Input: part model. Units: mm. Frame: model coordinates. Give positions to 0.01 mm unless a question says otherwise; leave off trailing zeros. Write each loop counter-clockwise with the first axis right and the second up, starting at its lowest first coordinate (ties: lowest second). Pieces come first, ordered by that corner, then holes. Notation, with made-up numbers: (33.5, 4.5) - (70.5, 4.5) arc R25 cw to (70.5, 35.5) - close; hole circle Ø8 at (65, -6). An arc over 180 degrees is marked (long way). Answer as CSV lines item,"result".
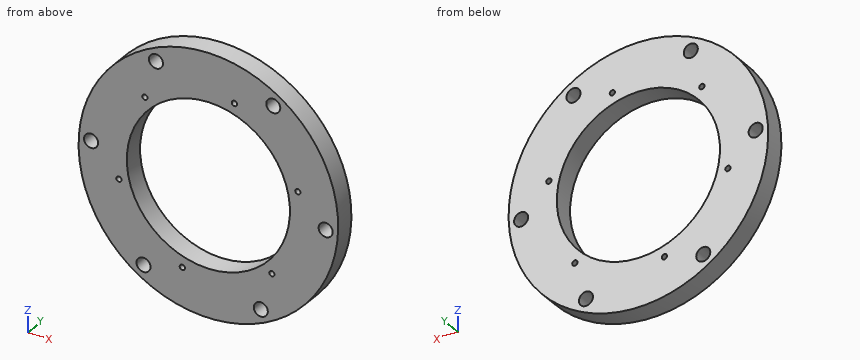
```python
from build123d import *

# Parameters (mm, degrees)
SKETCH_1_R      = 74
SKETCH_1_R_2    = 46.5
SKETCH_1_R_3    = 1.5
SKETCH_1_R_4    = 4
EXTRUDE_2_DEPTH = 12


with BuildPart() as part:
    # 草图1 → 凸台-拉伸2 (new body)
    with BuildSketch(Plane(origin=(0, 0, 0), x_dir=(1, 0, 0), z_dir=(0, 1, 0))):
        with Locations(Location((0, 0, 0), (0, 0, 270))):
            Circle(SKETCH_1_R)
        with Locations(Location((0, 0, 0), (0, 0, 270))):
            Circle(SKETCH_1_R_2, mode=Mode.SUBTRACT)
        with Locations(Location((36.199702934, 38.024091146, 0), (0, 0, 270))):
            Circle(SKETCH_1_R_3, mode=Mode.SUBTRACT)
        with Locations(Location((29.881416045, 59.967499324, 0), (0, 0, 270))):
            Circle(SKETCH_1_R_4, mode=Mode.SUBTRACT)
        with Locations(Location((66.874085838, 4.105684266, 0), (0, 0, 270))):
            Circle(SKETCH_1_R_4, mode=Mode.SUBTRACT)
        with Locations(Location((51.029680355, -12.337816778, 0), (0, 0, 270))):
            Circle(SKETCH_1_R_3, mode=Mode.SUBTRACT)
        with Locations(Location((36.992669793, -55.861815058, 0), (0, 0, 270))):
            Circle(SKETCH_1_R_4, mode=Mode.SUBTRACT)
        with Locations(Location((14.829977421, -50.361907923, 0), (0, 0, 270))):
            Circle(SKETCH_1_R_3, mode=Mode.SUBTRACT)
        with Locations(Location((-29.881416045, -59.967499324, 0), (0, 0, 270))):
            Circle(SKETCH_1_R_4, mode=Mode.SUBTRACT)
        with Locations(Location((-36.199702934, -38.024091146, 0), (0, 0, 270))):
            Circle(SKETCH_1_R_3, mode=Mode.SUBTRACT)
        with Locations(Location((-66.874085838, -4.105684266, 0), (0, 0, 270))):
            Circle(SKETCH_1_R_4, mode=Mode.SUBTRACT)
        with Locations(Location((-51.029680355, 12.337816778, 0), (0, 0, 270))):
            Circle(SKETCH_1_R_3, mode=Mode.SUBTRACT)
        with Locations(Location((-36.992669793, 55.861815058, 0), (0, 0, 270))):
            Circle(SKETCH_1_R_4, mode=Mode.SUBTRACT)
        with Locations(Location((-14.829977421, 50.361907923, 0), (0, 0, 270))):
            Circle(SKETCH_1_R_3, mode=Mode.SUBTRACT)
    extrude(amount=EXTRUDE_2_DEPTH)


solid = part.part
```
Item 1: Cut plane B-B on z = 43.5. Return the cut outline in (x, y), plus the area to 3 significant figures.
The answers:
outline,"(-59.86, 0) - (-16.43, 0) - (-16.43, 12) - (-59.86, 12) - close; (16.43, 0) - (59.86, 0) - (59.86, 12) - (16.43, 12) - close"
area,"1,040 mm²"
Item 2: Cut plane C-C on y = 3.75. Count the separate pieces of the cut face and the enclosed holes in it, plus the area to 3 significant figures.
The answers:
separate pieces,"1"
enclosed holes,"13"
area,"10,100 mm²"
Item 3: Contact query for flat-ended pins moving along their axis: pin 1 (13 mm diameter, centred on x = -36.99, z = -55.86, fed in from +Y); pin 2 (6.5 mm diameter, centred on x = 66.87, z = -4.11, fed in from -Y); pin 3 (1.5 mm diameter, centred on x = -57.5, y = 2, fed in from +Z); pin 4 (1.5 mm diameter, centred on y = 5.5, z = -48, fed in from +X). Output: stop coordinate, or through.
The answers:
pin 1,"y = 12"
pin 2,"through"
pin 3,"z = 47.49"
pin 4,"x = 56.95"
Item 4: Ray query, line 1 (Z direction, x = 1.5, y = 3.5); line 2 (Z direction, x = 28, y = 4.75); line 3 (X direction, y = 2.75, z = -6). Return the intervals inside material, ascending. Write a range as from..to.
The answers:
line 1,"-73.98..-46.48, 46.48..73.98"
line 2,"-68.5..-63.5, -56.44..-37.12, 37.12..68.5"
line 3,"-73.76..-46.11, 46.11..63.35, 70.4..73.76"
Item 5: Cut plane A-A on x = 0. Return the cut outline in (y, z).
The answers:
outline,"(0, -74) - (12, -74) - (12, -46.5) - (0, -46.5) - close; (0, 46.5) - (12, 46.5) - (12, 74) - (0, 74) - close"
Item 6: Cut plane D-D on x = -55.5. Return the cut outline in (y, z), plus the area to 3 significant figures.
The answers:
outline,"(0, -48.95) - (12, -48.95) - (12, 48.95) - (0, 48.95) - close"
area,"1,170 mm²"
